from build123d import *

# Parameters (mm, degrees)
BOSS_EXTRUDE1_DEPTH = 2
FILLET1_R           = 0.5
FILLET2_R           = 1


with BuildPart() as part:
    # Sketch1 → Boss-Extrude1 (new body)
    with BuildSketch(Plane.XY):
        with BuildLine():
            Line((-6.414814566, 10.280159843), (-5, 5))
            Line((-5, 5), (-5, -5))
            Line((-5, -5), (5, -5))
            Line((5, -5), (5, 5))
            Line((5, 5), (6.414814566, 10.280159843))
            ThreePointArc((6.414814566, 10.280159843), (6.374781392, 11.708496992), (5.558954759, 12.881602518))
            Line((5.558954759, 12.881602518), (4.965925826, 10.66838841))
            ThreePointArc((4.965925826, 10.66838841), (3.741180955, 9.961281629), (3.034074174, 11.1860265))
            Line((3.034074174, 11.1860265), (3.627103106, 13.399240608))
            ThreePointArc((3.627103106, 13.399240608), (2.334023755, 12.791214738), (1.585185434, 11.574255068))
            Line((1.585185434, 11.574255068), (0, 5.658262488))
            Line((0, 5.658262488), (-1.585185434, 11.574255068))
            ThreePointArc((-1.585185434, 11.574255068), (-2.334023755, 12.791214738), (-3.627103106, 13.399240608))
            Line((-3.627103106, 13.399240608), (-3.034074174, 11.1860265))
            ThreePointArc((-3.034074174, 11.1860265), (-3.741180955, 9.961281629), (-4.965925826, 10.66838841))
            Line((-4.965925826, 10.66838841), (-5.558954759, 12.881602518))
            ThreePointArc((-5.558954759, 12.881602518), (-6.374781392, 11.708496992), (-6.414814566, 10.280159843))
        make_face()
    extrude(amount=BOSS_EXTRUDE1_DEPTH)

    # Fillet1
    fillet1_edges = [part.edges().sort_by_distance(p)[0] for p in [
        (5.558954759, 12.881602518, 1),
        (-5.558954759, 12.881602518, 1),
        (-3.627103106, 13.399240608, 1),
        (3.627103106, 13.399240608, 1),
    ]]
    fillet(fillet1_edges, radius=FILLET1_R)

    # Fillet2
    fillet2_edges = [part.edges().sort_by_distance(p)[0] for p in [
        (0, 5.658262488, 1),
    ]]
    fillet(fillet2_edges, radius=FILLET2_R)


solid = part.part
CAD build for the part. Positions are in the model's coordinates, mm. A direction names the side the tool comes from. Give positions to 0.01 mm unless a question says otherwise; leave off trailing zeros. Loops run counter-clockwise (first coordinate to the right, second up) from the corner with the lowest first, then second, coordinate; pieces in that order, holes last. Notation, with made-up numbers: M 3.5,-30 L 38.5,-30 A35 cw 38.5,2 Z; hole C -26,-35.75 d11. An arc over 180 degrees is marked long. Write each question's results on one line, items separated by ' | '.
Q1. Band-saw the part on D-D on x = 4. Write the cut outline in (y, z).
Geometry check:
outline: M -5,0 L 9.93,0 L 9.93,2 L -5,2 Z
Q2. Band-saw the part on A-A on z = 1.15. Write the cut outline in (x, y).
Geometry check:
outline: M -6.41,10.28 L -5,5 L -5,-5 L 5,-5 L 5,5 L 6.41,10.28 A2.5 ccw 6.24,12.04 A0.5 ccw 5.31,11.95 L 4.97,10.67 A1 cw 3.03,11.19 L 3.38,12.46 A0.5 ccw 2.62,13.01 A2.5 ccw 1.59,11.57 L 0.97,9.26 A1 cw -0.97,9.26 L -1.59,11.57 A2.5 ccw -2.62,13.01 A0.5 ccw -3.38,12.46 L -3.03,11.19 A1 cw -4.97,10.67 L -5.31,11.95 A0.5 ccw -6.24,12.04 A2.5 ccw Z
Q3. Which spindle directions (+Z, -Z, +X, -X, +Y, -Y) get a long thin tool onto all of the face, cutting with end or side? Do faces 1 (the face through (5, 0, 1)), 2 (the face through (-1.27, 10.4, 0.99)), 3 (the face through (-3.2, 11.8, 1)). Say none if no direction does.
Geometry check:
face 1: +Z, -Z, +X, -Y | face 2: +Z, -Z, +Y | face 3: +Z, -Z
Q4. Flat gauge pins, fed straight in: P1, Ø2, axis at x = 0, y = 10.5, coming from the +Z side; P2, Ø1, axis at x = -3, z = 1.5, coming from the +Y side. Where does each tip first touch, or does it go through?
Geometry check:
P1: passes through | P2: stops at y = 13.09
Q5. Band-saw the part on B-B on y = 9.5. Write the cut outline in (x, z).
Geometry check:
outline: M -6.21,0 L -1.03,0 L -1.03,2 L -6.21,2 Z; M 1.03,0 L 6.21,0 L 6.21,2 L 1.03,2 Z
Q6. Band-saw the part on C-C on y = -2.25. Write the cut outline in (x, z), and give its area (3 significant figures).
Geometry check:
outline: M -5,0 L 5,0 L 5,2 L -5,2 Z | area: 20.0 mm²
Q7. Mould opens along X. For faces 4 (the face through (5.698, 7.603, 0.986)), 5 (the face through (-6.486, 11.188, 0.986)), 6 (the face through (0, 4, 0)), 7 (the face through (-1.963, 12.376, 0.986)) say: pulls with the +X half, pulls with the -X half, needs draft (parallel to the pull), parting line crosses it, or undercut.
Geometry check:
face 4: pulls with the +X half | face 5: pulls with the -X half | face 6: needs draft | face 7: undercut
Q8. Probe probe 1 along X at (y, z) = (10.5, 0.7); probe 2 along X at (y, z) = (11, 0.5); probe 3 along X at (y, z) = (2.75, 1.5). List the from-to ranges inside material, lowest first.
Geometry check:
probe 1: x = -6.46 to -4.9, -3.1 to -1.3, 1.3 to 3.1, 4.9 to 6.46 | probe 2: x = -6.5 to -5.05, -3 to -1.43, 1.43 to 3, 5.05 to 6.5 | probe 3: x = -5 to 5
